Input: dimensioned drawing with shaded views. Units: mm. Origin: part minimum x, y, z. Coordinates: 2 decimals unless noted, no trailing zeros. Order: outer loops, then holes, each group sorted by start corner. A loop starts at its lowest first (then second) coordinate and runs counter-clockwise, first axis right, second up. Notation, with made-up numbers: (29.5, -16) -> (87.5, -16) arc R16 ccw to (87.5, -8) -> close; hole circle Ø3 at (-37.75, 45). An arc over 180 degrees is marked (long way). Put each result on its own line as item: value.
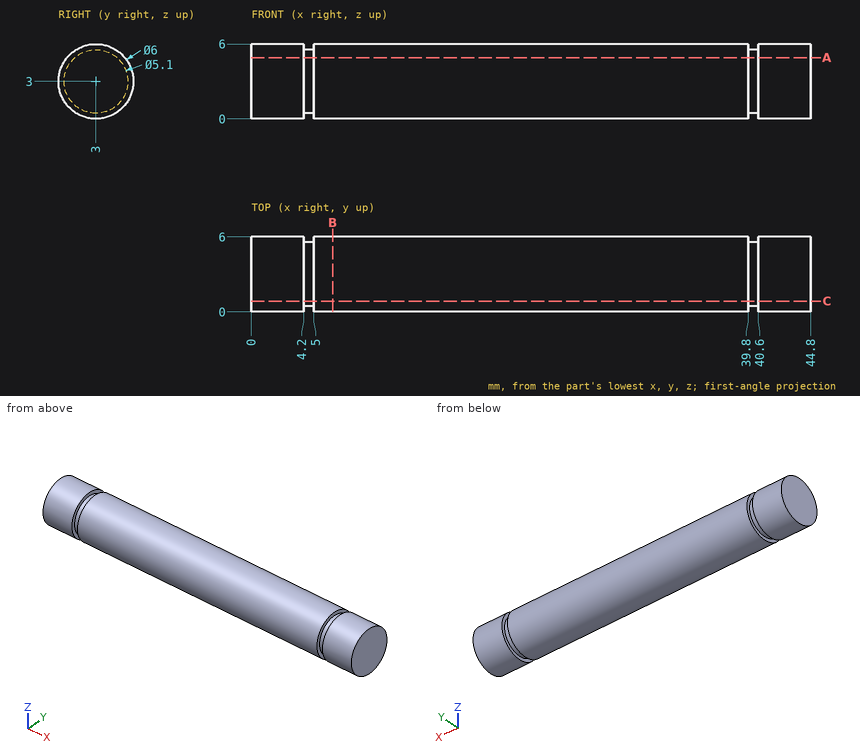
1. Ray query, line 1 along X through (y, z) = (4.6, 5.35); line 2 along Y through (x, z) = (24, 3.2); line 3 along Y through (x, z) = (23, 5.4). Return the intervals inside material, ascending.
Numbers:
line 1: x = 0 to 4.2, 5 to 39.8, 40.6 to 44.8
line 2: y = 0.01 to 5.99
line 3: y = 1.2 to 4.8
2. Cut plane A-A on z = 4.9. Output: boundary loops of the cut face in (x, y).
Numbers:
outline: (0, 0.68) -> (4.2, 0.68) -> (4.2, 1.3) -> (5, 1.3) -> (5, 0.68) -> (39.8, 0.68) -> (39.8, 1.3) -> (40.6, 1.3) -> (40.6, 0.68) -> (44.8, 0.68) -> (44.8, 5.32) -> (40.6, 5.32) -> (40.6, 4.7) -> (39.8, 4.7) -> (39.8, 5.32) -> (5, 5.32) -> (5, 4.7) -> (4.2, 4.7) -> (4.2, 5.32) -> (0, 5.32) -> close
3. Cut plane B-B on x = 6.5. Output: boundary loops of the cut face in (y, z), plus the area to 3 significant figures.
Numbers:
outline: circle Ø6 at (3, 3)
area: 28.3 mm2
4. Cut plane C-C on y = 0.85. Output: boundary loops of the cut face in (x, z).
Numbers:
outline: (0, 0.91) -> (4.2, 0.91) -> (4.2, 1.63) -> (5, 1.63) -> (5, 0.91) -> (39.8, 0.91) -> (39.8, 1.63) -> (40.6, 1.63) -> (40.6, 0.91) -> (44.8, 0.91) -> (44.8, 5.09) -> (40.6, 5.09) -> (40.6, 4.37) -> (39.8, 4.37) -> (39.8, 5.09) -> (5, 5.09) -> (5, 4.37) -> (4.2, 4.37) -> (4.2, 5.09) -> (0, 5.09) -> close
